Input: part model. Units: mm. Frame: model coordinates. Face numbers are marked on the shaded views. A direction names the side the tool comes from. Coordinates: 2 decimals unless noted, no trailing zeros. Write each loop counter-clockwise with the first axis right and the second up, starting at its lowest first coordinate (ties: lowest second). Pieces come first, ordered by that corner, then holes. Notation, with made-up numbers: (37, 85) - (92, 85) arc R29 cw to (92, 112) - close; hole circle Ø10 at (-35.5, 59). An arc over 180 degrees is marked (long way). Use a Markdown table: item, result. Add a question column.
Q1. Section query D-D (z = 22). Return the cut outline in (x, y).
Q2. Mould query, pull axis X, two halves, no side actions, for the marked faces 1, 2 and 3. Classes: released by +X, released by -X, zero draft, split by the parting line, or undercut.
Q3. Material intervals for probe 1 along X at (y, z) = (-41.5, 24.5); probe 2 along X at (y, z) = (-37, 27.5); probe 3 along X at (y, z) = (-65, 49.5), sorted ascending. Write a range as from..to.
Q4. Set-up query: the marked faces 4, 5, 6, 7 and 8. Return all of +Z, -Z, +X, -X, +Y, -Y with unobstructed straight access to the full face (end or side cutting, diameter ignored); none if empty.
Q5. Section query B-B (y = -50.5). Return the cut outline in (x, z), then the cut area to 3 significant figures.
Q6. Section query A-A (z = 9). Return the cut outline in (x, y).
Q7. Section query C-C (z = 42). Return the cut outline in (x, y).
Q8. Pin query (flat end, axial travel): P1, Ø2, axis at y = -13, z = 39.5, coming from the -X side; P2, Ø4, axis at x = 12, y = -27.5, coming from the -Z side; P3, Ø2, axis at y = -14.5, z = 33.5, coming from the -X side. Return the tip coordinate at first contact, or that it passes through.
from build123d import *

# Parameters (mm, degrees)
F1_DEPTH = 76.2


with BuildPart() as f1:
    # F0 (on Front) → F1 (new body)
    with BuildSketch(Plane.XZ):
        Polygon((-44.533051, 10.691937), (-27.366411, 0), (-23.028744, 6.964423), (-33.808812, 13.678597), (-27.366411, 24.022314), (-33.752983, 28.000077), align=None)
        Polygon((40.3336, 82.164579), (25.692132, 58.656697), (25.692132, 0), (40.3336, 0), align=None)
        Polygon((-23.028744, 6.964423), (-27.366411, 0), (-10.841151, 0), (25.692132, 58.656697), (40.3336, 82.164579), (28.427108, 89.580327), align=None)
    extrude(amount=F1_DEPTH)


solid = f1.part
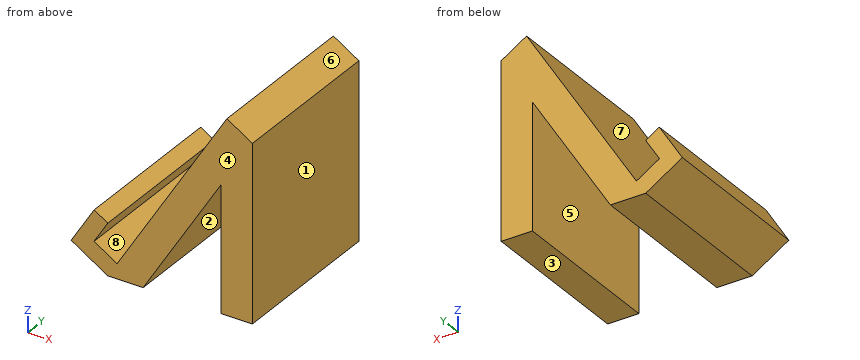
Values follow:
| question | item | result |
|---|---|---|
| 1 | outline | (-37.49, -76.2) - (-28.63, -76.2) - (-28.63, 0) - (-37.49, 0) - close; (-13.66, -76.2) - (2.86, -76.2) - (2.86, 0) - (-13.66, 0) - close; (25.69, -76.2) - (40.33, -76.2) - (40.33, 0) - (25.69, 0) - close |
| 2 | face 1 | released by +X |
| 2 | face 2 | undercut |
| 2 | face 3 | zero draft |
| 3 | probe 1 | -35.93..-28.13, -12.11..4.42, 25.69..40.33 |
| 3 | probe 2 | -34.06..-32.95, -10.24..6.29, 25.69..40.33 |
| 3 | probe 3 | 3.46..19.99, 25.69..40.33 |
| 4 | face 4 | +Z, -Z, +X, -X, -Y |
| 4 | face 5 | -Z, +Y, -Y |
| 4 | face 6 | +Z, +X, +Y, -Y |
| 4 | face 7 | +Z, +Y, -Y |
| 4 | face 8 | +Y, -Y |
| 5 | outline | (-44.53, 10.69) - (-27.37, 0) - (-10.84, 0) - (25.69, 58.66) - (25.69, 0) - (40.33, 0) - (40.33, 82.16) - (28.43, 89.58) - (-23.03, 6.96) - (-33.81, 13.68) - (-27.37, 24.02) - (-33.75, 28) - close |
| 5 | area | 2,710 mm2 |
| 6 | outline | (-41.82, -76.2) - (-26.3, -76.2) - (-26.3, 0) - (-41.82, 0) - close; (-21.76, -76.2) - (-5.24, -76.2) - (-5.24, 0) - (-21.76, 0) - close; (25.69, -76.2) - (40.33, -76.2) - (40.33, 0) - (25.69, 0) - close |
| 7 | outline | (-1.21, -76.2) - (15.32, -76.2) - (15.32, 0) - (-1.21, 0) - close; (25.69, -76.2) - (40.33, -76.2) - (40.33, 0) - (25.69, 0) - close |
| 8 | P1 | x = -3.39 |
| 8 | P2 | z = 33.46 |
| 8 | P3 | x = -7.12 |
